Could you check a few things on this model? Use its own coordinates, in mm. A direction names the side the tool comes from. Coordinates: 2 decimals unless noted, no trailing zeros. Loops run counter-clockwise (first coordinate to the right, second up) from the corner with the lowest first, then second, coordinate; pieces in that order, holes last. Notation, with made-up numbers: (66.5, 60.25) - (96.5, 60.25) arc R34 ccw to (96.5, 98.25) - close; hole circle Ø8 at (-21.5, 89). An arc over 180 degrees is marked (long way). Put each result on its own line as item: value. Start each with the question number.
```python
from build123d import *

# Parameters (mm, degrees)
SZKIC1_W                       = 42
SZKIC1_H                       = 54
SZKIC1_R                       = 14
DODANIE_WYCI_GNI_CIE1_DEPTH    = 38
SFAZOWANIE1_SIZE               = 1
OTW_R_GWINTOWANY_M6X1_01_D     = 5
OTW_R_GWINTOWANY_M6X1_01_DEPTH = 17
OTW_R_GWINTOWANY_M6X1_01_TIP   = 1.502151548
OTW_R_GWINTOWANY_M5X0_81_D     = 4.2
OTW_R_GWINTOWANY_M5X0_81_DEPTH = 25
OTW_R_GWINTOWANY_M5X0_81_TIP   = 1.2618073
SFAZOWANIE2_SIZE               = 10


with BuildPart() as part:
    # Szkic1 → Dodanie-wyciągnięcie1 (new body)
    with BuildSketch(Plane.XY):
        with Locations((21, 27)):
            Rectangle(SZKIC1_W, SZKIC1_H)
        with Locations((20.5, 27)):
            Circle(SZKIC1_R, mode=Mode.SUBTRACT)
    extrude(amount=DODANIE_WYCI_GNI_CIE1_DEPTH)

    # Sfazowanie1
    sfazowanie1_edges = [part.edges().sort_by_distance(p)[0] for p in [
        (6.5, 27, 0),
        (6.5, 27, 38),
    ]]
    chamfer(sfazowanie1_edges, length=SFAZOWANIE1_SIZE)

    # Otwór gwintowany M6x1.01
    with Locations(Plane.XY.offset(38)):
        with Locations((33.935028843, 40.435028843), (7.064971157, 40.435028843), (7.064971157, 13.564971157), (33.935028843, 13.564971157)):
            Hole(OTW_R_GWINTOWANY_M6X1_01_D / 2, depth=OTW_R_GWINTOWANY_M6X1_01_DEPTH)
            with Locations((0, 0, -(OTW_R_GWINTOWANY_M6X1_01_DEPTH + OTW_R_GWINTOWANY_M6X1_01_TIP / 2))):  # 118° drill point
                Cone(0, OTW_R_GWINTOWANY_M6X1_01_D / 2, OTW_R_GWINTOWANY_M6X1_01_TIP, mode=Mode.SUBTRACT)

    # Otwór gwintowany M5x0.81
    with Locations(Plane(origin=(42, 0, 0), x_dir=(0, 0, -1), z_dir=(1, 0, 0))):
        with Locations((-32, 48), (-6, 48), (-6, 6), (-32, 6)):
            Hole(OTW_R_GWINTOWANY_M5X0_81_D / 2, depth=OTW_R_GWINTOWANY_M5X0_81_DEPTH)
            with Locations((0, 0, -(OTW_R_GWINTOWANY_M5X0_81_DEPTH + OTW_R_GWINTOWANY_M5X0_81_TIP / 2))):  # 118° drill point
                Cone(0, OTW_R_GWINTOWANY_M5X0_81_D / 2, OTW_R_GWINTOWANY_M5X0_81_TIP, mode=Mode.SUBTRACT)

    # Sfazowanie2
    sfazowanie2_edges = [part.edges().sort_by_distance(p)[0] for p in [
        (0, 54, 19),
        (0, 0, 19),
    ]]
    chamfer(sfazowanie2_edges, length=SFAZOWANIE2_SIZE)


solid = part.part
```
(1) For pin 1 Ø4 at (y, z) = (48, 32) entering from +X; pin 2 Ø5 at (y, z) = (6, 6) entering from -X; pin 3 Ø4 at (y, z) = (48, 6) entering from -X, each with a flat end and sliding along its axis, tell me the tip position at first contact or that it passes through.
(2) I want a section at A-A on x = 20.5. List the corners of the cut face in (y, z) for me, and give its area (3 significant figures).
(3) Which directions (+Z, -Z, +X, -X, +Y, -Y) give clear straight access to the entire face, cutting with the end or side of a thin tool? Please do faces 5 (the cylindrical face through (5.721, 42.543, 29.381)), 6 (the conical face through (15.96, 48.25, 6.27)).
(4) I need wall thicknesses on L1, parallel to Z at x = 34, y = 48; L2, parallel to Y at x = 20.5, z = 14; L3, parallel to X at y = 14.5, z = 20.5. Which ranges of each line are inside material? Lowest first, please. Write a range as [from, to].
(5) If we mould it in two halves opening along Z, with no side actions, what happens to faces 1 (the cylindrical face through (29.325, 46.722, 30.334)), 2 (the flat face through (35, 21, 0)), 3 (the cylindrical face through (29.33, 45.95, 5.54)), 4 (the cylindrical face through (4.756, 12.607, 29.381))? For each: pulls with the +Z half, pulls with the -Z half, needs draft (parallel to the pull), parting line crosses it, or undercut.
(6) I want a section at C-C on x = 37.5. List the corners of the cut face in (y, z) for me, and give its area (3 significant figures).
(7) I want a section at D-D on z = 35.5. List the corners of the cut face in (x, y) for me, and give its area (3 significant figures).
(8) I want a section at B-B on y = 27. List the corners of the cut face in (x, z) for me, and give its area (3 significant figures).
Answer sheet:
1. pin 1: stops at x = 16.94
1. pin 2: stops at x = 1.5
1. pin 3: stops at x = 2
2. outline: (0, 0) - (12, 0) - (13, 1) - (13, 37) - (12, 38) - (0, 38) - close; (41, 1) - (42, 0) - (54, 0) - (54, 38) - (42, 38) - (41, 37) - close; hole circle Ø4.2 at (6, 6); hole circle Ø4.2 at (6, 32); hole circle Ø4.2 at (48, 6); hole circle Ø4.2 at (48, 32)
2. area: 931 mm^2
3. face 5: +Z
3. face 6: +X
4. L1: z = [0, 3.9], [8.1, 29.9], [34.1, 38]
4. L2: y = [0, 13], [41, 54]
4. L3: x = [0, 5.68], [8.45, 14.2], [26.8, 32.55], [35.32, 42]
5. face 1: undercut
5. face 2: pulls with the -Z half
5. face 3: undercut
5. face 4: needs draft
6. outline: (0, 0) - (54, 0) - (54, 38) - (0, 38) - close; hole circle Ø4.2 at (6, 6); hole circle Ø4.2 at (6, 32); hole circle Ø4.2 at (48, 6); hole circle Ø4.2 at (48, 32)
6. area: 2,000 mm^2
7. outline: (0, 10) - (10, 0) - (42, 0) - (42, 54) - (10, 54) - (0, 44) - close; hole circle Ø5 at (7.06, 13.56); hole circle Ø5 at (7.06, 40.44); hole circle Ø28 at (20.5, 27); hole circle Ø5 at (33.94, 13.56); hole circle Ø5 at (33.94, 40.44)
7. area: 1,470 mm^2
8. outline: (0, 0) - (5.5, 0) - (6.5, 1) - (6.5, 37) - (5.5, 38) - (0, 38) - close; (34.5, 1) - (35.5, 0) - (42, 0) - (42, 38) - (35.5, 38) - (34.5, 37) - close
8. area: 530 mm^2
